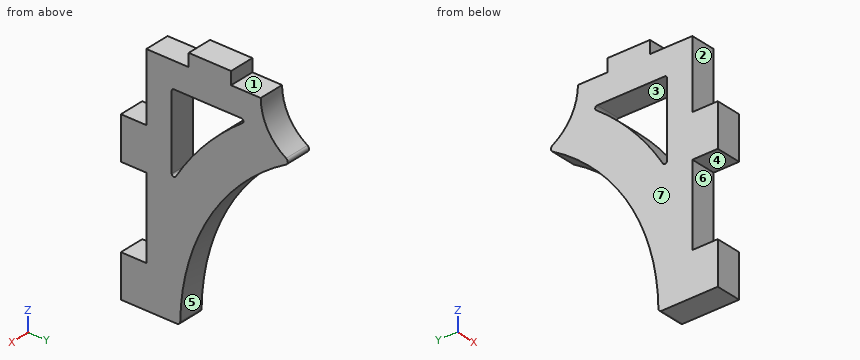
Autodesk Inventor part; units mm, degrees
ref_plane "YZ Plane" through (0, 0, 0) normal (1, 0, 0) x (0, 1, 0)
ref_plane "XZ Plane" through (0, 0, 0) normal (0, 1, 0) x (-1, 0, 0)
ref_plane "XY Plane" through (0, 0, 0) normal (0, 0, 1) x (1, 0, 0)
sketch "Sketch1" plane through (0, 0, 0) normal (1, 0, 0) x (0, 1, 0)
  circle A0 centre (-8.4812, -1.44) radius 50 construction
  line L0 (-46.4812, 56.56) -> (-56.4812, 56.56)
  line L1 (-56.4812, 56.56) -> (-56.4812, 53.56)
  line L2 (-66.4812, 27.56) -> (-72.4812, 27.56)
  line L3 (-72.4812, 27.56) -> (-72.4812, 37.56)
  line L4 (-72.4812, 37.56) -> (-66.4812, 37.56)
  arc A1 (-44.3506, 33.3937) -> (-32.2509, 42.5487) centre (-8.4812, -1.44) ccw construction
  line L5 (-66.4812, 53.56) -> (-66.4812, 37.56)
  line L6 (-56.4812, 53.56) -> (-66.4812, 53.56)
  line L7 (-66.4812, 53.56) -> (-45.3047, 32.3835) construction
  line L8 (-58.4812, -1.44) -> (-65.4812, -1.44)
  line L9 (-65.4812, -1.44) -> (-72.4812, -1.44)
  line L10 (-72.4812, -1.44) -> (-72.4812, 8.56)
  line L11 (-72.4812, 8.56) -> (-66.4812, 8.56)
  line L12 (-66.4812, 27.56) -> (-66.4812, 8.56)
  arc A2 (-32.2509, 42.5487) -> (-58.4812, -1.44) centre (-8.4812, -1.44) ccw
  arc A3 (-39.4812, 53.56) -> (-32.2509, 42.5487) centre (-27.4812, 53.56) ccw
  line L13 (-46.4812, 56.56) -> (-46.4812, 53.56)
  line L14 (-46.4812, 53.56) -> (-39.4812, 53.56)
  line L15 (-48.4406, 53.56) -> (-18.7746, 53.56) construction
  point P0 (-30.5194, 43.4412)
  dimension "d6" = 50
  dimension "d8" = 10
  dimension "d10" = 3
  dimension "d11" = 10
  dimension "d12" = 6
  dimension "d18" = 10
  dimension "d23" = 45
  dimension "d30" = 10
  dimension "d31" = 6
  dimension "d32" = 19
  dimension "d38" = 58
  dimension "d50" = 7
  dimension "d51" = 16
  dimension "d57" = 12
  dimension "d69" = 7
  dimension "d70" = 7
extrude "Extrusion2" add sketch "Sketch1" along normal blind 6
fillet "Fillet3" radius 0.75 2 edges at (3, -32.2509, 42.5487) (3, -58.4812, -1.44)
sketch "Sketch2" plane through (6, 0, 0) normal (1, 0, 0) x (0, 0, -1)
  line L0 (-27.7662, -60.4812) -> (-47.56, -60.4812)
  line L1 (-47.56, -60.4812) -> (-47.56, -42.4812)
  line L2 (-53.56, -56.4812) -> (-53.56, -66.4812)
  line L3 (-53.56, -66.4812) -> (-37.56, -66.4812)
  line L4 (-56.56, -46.4812) -> (-56.56, -56.4812)
  arc A0 (-41.8649, -33.4749) -> (0.701, -58.4757) centre (1.44, -8.4812) ccw
  arc A1 (-47.56, -42.4812) -> (-27.7662, -60.4812) centre (1.44, -8.4812) ccw
  point P0 (-53.56, -39.4812)
  dimension "d42" = 6
  dimension "d43" = 6
  dimension "d73" = 3
extrude "Extrusion5" cut sketch "Sketch2" against normal blind 10
fillet "Fillet7" radius 0.5 3 edges at (3, -42.4812, 47.56) (3, -60.4812, 47.56) (3, -60.4812, 27.7662)
properties part number "Harness Pusher 2"
Geometry check sheet. Reference: the model listing, model coordinates, mm. Face numbers are marked on the shaded views. A direction names the side the tool comes from. Round coordinates to 2 decimals unless told otherwise and drop trailing zeros. Order: outer loops, then holes, each group sorted by start corner. A loop starts at its lowest first (then second) coordinate and runs counter-clockwise, first axis right, second up. Notation, with made-up numbers: M 10.5,55 L 41.5,55 A22 cw 41.5,62 Z; hole C 57.25,27.25 d9. An arc over 180 degrees is marked long. Answer as CSV lines item,"result".
1) Sectioned sample at C-C on z = 10. Record the cut outline in (x, y), and give its area (3 significant figures).
Entries:
outline,"M 0,-66.48 L 6,-66.48 L 6,-57.15 L 0,-57.15 Z"
area,"56.0 mm2"
2) Gauge pin test, flat ends, axial feed: pin 1 Ø1.5 at (x, y) = (1.5, -40.5) entering from -Z; pin 2 Ø1.8 at (x, z) = (3, 19.5) entering from -Y; pin 3 Ø3 at (x, z) = (1.5, 46.5) entering from +Y. Record the tip position at first contact, or that the pin passes through.
Entries:
pin 1,"z = 36.33"
pin 2,"y = -66.48"
pin 3,"y = -35.89"
3) Sectioned sample at B-B on y = -51. Record the cut outline in (x, z), and give its area (3 significant figures).
Entries:
outline,"M 0,24.87 L 6,24.87 L 6,40.38 L 0,40.38 Z; M 0,47.56 L 6,47.56 L 6,56.56 L 0,56.56 Z"
area,"147 mm2"
4) Tool access check on the marked faces 1, 2 and 3. Record the directions out of +Z, -Z, +X, -X, +Y, -Y that give a thin tool (end or side, any length) a straight path to the whole face; none if there is none.
Entries:
face 1,"+Z, +X, -X, +Y"
face 2,"+Z, +X, -X, -Y"
face 3,"+X, -X"
5) Thickness scan on probe 1 along Z at (x, y) = (5, -71); probe 2 along Z at (x, y) = (1.5, -60); probe 3 along Y at (x, z) = (1.75, 30.5). Record the ranges inside material, lowest first. Write a range as [from, to].
Entries:
probe 1,"[-1.44, 8.56], [27.56, 37.56]"
probe 2,"[-1.44, 29.12], [47.56, 53.56]"
probe 3,"[-72.48, -60.48], [-58.85, -46.95]"
6) Sectioned sample at D-D on y = -37.5. Record the cut outline in (x, z).
Entries:
outline,"M 0,39.28 L 6,39.28 L 6,46.96 L 0,46.96 Z"
7) Sectioned sample at A-A on y = -69. Record the cut outline in (x, z).
Entries:
outline,"M 0,-1.44 L 6,-1.44 L 6,8.56 L 0,8.56 Z; M 0,27.56 L 6,27.56 L 6,37.56 L 0,37.56 Z"
8) Mould release check, pull along Z, two halves, no side actions. Record for the marked faces 4, 5, 6 and 7: +Z half, -Z half, draft (parallel to the pull), parting line (faces both ways), or undercut.
Entries:
face 4,"undercut"
face 5,"-Z half"
face 6,"undercut"
face 7,"draft"
